```python
from build123d import *

# Parameters (mm, degrees)
PAD_DEPTH        = 1
POCKET_DEPTH     = 0.001
HOLE_D           = 1.75
HOLE_CSINK_D     = 3.3
HOLE_CSINK_ANGLE = 90
SKETCH025_R      = 5.25
SKETCH025_R_2    = 1.5
POCKET007_DEPTH  = 5
POCKET008_DEPTH  = 1.001
POCKET010_DEPTH  = 5
POCKET011_DEPTH  = 1.001


with BuildPart() as part:
    # Sketch → Pad (new body)
    with BuildSketch(Plane.XY):
        with BuildLine():
            Line((-51.8, 52.175), (51.8, 52.175))
            ThreePointArc((52.175, 51.8), (52.065165, 52.065165), (51.8, 52.175))
            Line((52.175, 51.8), (52.175, -51.8))
            ThreePointArc((51.8, -52.175), (52.065165, -52.065165), (52.175, -51.8))
            Line((51.8, -52.175), (-51.8, -52.175))
            ThreePointArc((-52.175, -51.8), (-52.065165, -52.065165), (-51.8, -52.175))
            Line((-52.175, -51.8), (-52.175, 51.8))
            ThreePointArc((-51.8, 52.175), (-52.065165, 52.065165), (-52.175, 51.8))
        make_face()
    extrude(amount=-PAD_DEPTH)

    # Sketch002 → Pocket (cut, through all)
    with BuildSketch(Plane.XY.offset(-4.8)):
        with BuildLine():
            Line((-45, 50.175), (45, 50.175))
            ThreePointArc((45, 50.175), (45.353553, 50.321447), (45.5, 50.675))
            ThreePointArc((45.5, 50.675), (45.353553, 51.028553), (45, 51.175))
            Line((-45, 51.175), (45, 51.175))
            ThreePointArc((-45, 51.175), (-45.353553, 51.028553), (-45.5, 50.675))
            ThreePointArc((-45.5, 50.675), (-45.353553, 50.321447), (-45, 50.175))
        make_face()
        with BuildLine():
            Line((-45, -51.175), (45, -51.175))
            ThreePointArc((45, -51.175), (45.353553, -51.028553), (45.5, -50.675))
            ThreePointArc((45.5, -50.675), (45.353553, -50.321447), (45, -50.175))
            Line((-45, -50.175), (45, -50.175))
            ThreePointArc((-45, -50.175), (-45.353553, -50.321447), (-45.5, -50.675))
            ThreePointArc((-45.5, -50.675), (-45.353553, -51.028553), (-45, -51.175))
        make_face()
        with BuildLine():
            Line((51.175, -45), (51.175, 45))
            ThreePointArc((51.175, 45), (51.028553, 45.353553), (50.675, 45.5))
            ThreePointArc((50.675, 45.5), (50.321447, 45.353553), (50.175, 45))
            Line((50.175, -45), (50.175, 45))
            ThreePointArc((50.175, -45), (50.321447, -45.353553), (50.675, -45.5))
            ThreePointArc((50.675, -45.5), (51.028553, -45.353553), (51.175, -45))
        make_face()
        with BuildLine():
            Line((-50.175, -45), (-50.175, 45))
            ThreePointArc((-50.175, 45), (-50.321447, 45.353553), (-50.675, 45.5))
            ThreePointArc((-50.675, 45.5), (-51.028553, 45.353553), (-51.175, 45))
            Line((-51.175, -45), (-51.175, 45))
            ThreePointArc((-51.175, -45), (-51.028553, -45.353553), (-50.675, -45.5))
            ThreePointArc((-50.675, -45.5), (-50.321447, -45.353553), (-50.175, -45))
        make_face()
    extrude(amount=-POCKET_DEPTH, mode=Mode.SUBTRACT)

    # Hole (through all)
    with Locations(Plane.XY):
        with Locations((-50, 50), (50, 50), (50, -50), (-50, -50)):
            CounterSinkHole(HOLE_D / 2, HOLE_CSINK_D / 2, counter_sink_angle=HOLE_CSINK_ANGLE)

    # Sketch025 → Pocket007 (cut)
    with BuildSketch(Plane.XY):
        with Locations((26.67, 26.67)):
            Circle(SKETCH025_R)
        with Locations((5.824921, 36.39022)):
            Circle(SKETCH025_R_2)
        with Locations((7.829503, 39.862258)):
            Circle(SKETCH025_R_2)
        with Locations((10.406544, 42.933456)):
            Circle(SKETCH025_R_2)
        with Locations((13.477742, 45.510497)):
            Circle(SKETCH025_R_2)
        with Locations((16.94978, 47.515079)):
            Circle(SKETCH025_R_2)
    extrude(amount=-POCKET007_DEPTH, mode=Mode.SUBTRACT)

    # Sketch027 → Pocket008 (cut, through all)
    with BuildSketch(Plane.XY):
        with BuildLine():
            Line((-49.17, 11.27), (-49.17, 42.07))
            ThreePointArc((-47.17, 44.07), (-48.584214, 43.484214), (-49.17, 42.07))
            Line((-47.17, 44.07), (-6.17, 44.07))
            ThreePointArc((-4.17, 42.07), (-4.755786, 43.484214), (-6.17, 44.07))
            Line((-4.17, 42.07), (-4.17, 11.27))
            ThreePointArc((-6.17, 9.27), (-4.755786, 9.855786), (-4.17, 11.27))
            Line((-6.17, 9.27), (-47.17, 9.27))
            ThreePointArc((-49.17, 11.27), (-48.584214, 9.855786), (-47.17, 9.27))
        make_face()
    extrude(amount=-POCKET008_DEPTH, mode=Mode.SUBTRACT)

    # Sketch029 → Pocket010 (cut)
    with BuildSketch(Plane.XY):
        with BuildLine():
            ThreePointArc((-33.17, 6.27), (-34.67, 4.77), (-33.17, 3.27))
            Line((-33.17, 3.27), (-30.17, 3.27))
            ThreePointArc((-30.17, 3.27), (-28.67, 4.77), (-30.17, 6.27))
            Line((-30.17, 6.27), (-33.17, 6.27))
        make_face()
        with BuildLine():
            ThreePointArc((-23.17, 6.27), (-24.67, 4.77), (-23.17, 3.27))
            Line((-23.17, 3.27), (-20.17, 3.27))
            ThreePointArc((-20.17, 3.27), (-18.67, 4.77), (-20.17, 6.27))
            Line((-20.17, 6.27), (-23.17, 6.27))
        make_face()
        with BuildLine():
            ThreePointArc((-13.17, 6.27), (-14.67, 4.77), (-13.17, 3.27))
            Line((-13.17, 3.27), (-10.17, 3.27))
            ThreePointArc((-10.17, 3.27), (-8.67, 4.77), (-10.17, 6.27))
            Line((-10.17, 6.27), (-13.17, 6.27))
        make_face()
        with BuildLine():
            ThreePointArc((-43.17, 6.27), (-44.67, 4.77), (-43.17, 3.27))
            Line((-43.17, 3.27), (-40.17, 3.27))
            ThreePointArc((-40.17, 3.27), (-38.67, 4.77), (-40.17, 6.27))
            Line((-40.17, 6.27), (-43.17, 6.27))
        make_face()
    extrude(amount=-POCKET010_DEPTH, mode=Mode.SUBTRACT)

    # Sketch030 → Pocket011 (cut, through all)
    with BuildSketch(Plane.XY):
        with BuildLine():
            Line((-48.505, -19.735), (-48.505, -6.935))
            ThreePointArc((-46.405, -4.835), (-47.889924, -5.450076), (-48.505, -6.935))
            Line((-46.405, -4.835), (-33.605, -4.835))
            ThreePointArc((-31.505, -6.935), (-32.120076, -5.450076), (-33.605, -4.835))
            Line((-31.505, -6.935), (-31.505, -19.735))
            ThreePointArc((-33.605, -21.835), (-32.120076, -21.219924), (-31.505, -19.735))
            Line((-33.605, -21.835), (-46.405, -21.835))
            ThreePointArc((-48.505, -19.735), (-47.889924, -21.219924), (-46.405, -21.835))
        make_face()
        with BuildLine():
            Line((-21.835, -19.735), (-21.835, -6.935))
            ThreePointArc((-19.735, -4.835), (-21.219924, -5.450076), (-21.835, -6.935))
            Line((-19.735, -4.835), (-6.935, -4.835))
            ThreePointArc((-4.835, -6.935), (-5.450076, -5.450076), (-6.935, -4.835))
            Line((-4.835, -6.935), (-4.835, -19.735))
            ThreePointArc((-6.935, -21.835), (-5.450076, -21.219924), (-4.835, -19.735))
            Line((-6.935, -21.835), (-19.735, -21.835))
            ThreePointArc((-21.835, -19.735), (-21.219924, -21.219924), (-19.735, -21.835))
        make_face()
        with BuildLine():
            Line((4.835, -19.735), (4.835, -6.935))
            ThreePointArc((6.935, -4.835), (5.450076, -5.450076), (4.835, -6.935))
            Line((6.935, -4.835), (19.735, -4.835))
            ThreePointArc((21.835, -6.935), (21.219924, -5.450076), (19.735, -4.835))
            Line((21.835, -6.935), (21.835, -19.735))
            ThreePointArc((19.735, -21.835), (21.219924, -21.219924), (21.835, -19.735))
            Line((19.735, -21.835), (6.935, -21.835))
            ThreePointArc((4.835, -19.735), (5.450076, -21.219924), (6.935, -21.835))
        make_face()
        with BuildLine():
            Line((31.505, -19.735), (31.505, -6.935))
            ThreePointArc((33.605, -4.835), (32.120076, -5.450076), (31.505, -6.935))
            Line((33.605, -4.835), (46.405, -4.835))
            ThreePointArc((48.505, -6.935), (47.889924, -5.450076), (46.405, -4.835))
            Line((48.505, -6.935), (48.505, -19.735))
            ThreePointArc((46.405, -21.835), (47.889924, -21.219924), (48.505, -19.735))
            Line((46.405, -21.835), (33.605, -21.835))
            ThreePointArc((31.505, -19.735), (32.120076, -21.219924), (33.605, -21.835))
        make_face()
        with BuildLine():
            Line((31.505, -46.405), (31.505, -33.605))
            ThreePointArc((33.605, -31.505), (32.120076, -32.120076), (31.505, -33.605))
            Line((33.605, -31.505), (46.405, -31.505))
            ThreePointArc((48.505, -33.605), (47.889924, -32.120076), (46.405, -31.505))
            Line((48.505, -33.605), (48.505, -46.405))
            ThreePointArc((46.405, -48.505), (47.889924, -47.889924), (48.505, -46.405))
            Line((46.405, -48.505), (33.605, -48.505))
            ThreePointArc((31.505, -46.405), (32.120076, -47.889924), (33.605, -48.505))
        make_face()
        with BuildLine():
            Line((4.835, -46.405), (4.835, -33.605))
            ThreePointArc((6.935, -31.505), (5.450076, -32.120076), (4.835, -33.605))
            Line((6.935, -31.505), (19.735, -31.505))
            ThreePointArc((21.835, -33.605), (21.219924, -32.120076), (19.735, -31.505))
            Line((21.835, -33.605), (21.835, -46.405))
            ThreePointArc((19.735, -48.505), (21.219924, -47.889924), (21.835, -46.405))
            Line((19.735, -48.505), (6.935, -48.505))
            ThreePointArc((4.835, -46.405), (5.450076, -47.889924), (6.935, -48.505))
        make_face()
        with BuildLine():
            Line((-21.835, -46.405), (-21.835, -33.605))
            ThreePointArc((-19.735, -31.505), (-21.219924, -32.120076), (-21.835, -33.605))
            Line((-19.735, -31.505), (-6.935, -31.505))
            ThreePointArc((-4.835, -33.605), (-5.450076, -32.120076), (-6.935, -31.505))
            Line((-4.835, -33.605), (-4.835, -46.405))
            ThreePointArc((-6.935, -48.505), (-5.450076, -47.889924), (-4.835, -46.405))
            Line((-6.935, -48.505), (-19.735, -48.505))
            ThreePointArc((-21.835, -46.405), (-21.219924, -47.889924), (-19.735, -48.505))
        make_face()
        with BuildLine():
            Line((-48.505, -46.405), (-48.505, -33.605))
            ThreePointArc((-46.405, -31.505), (-47.889924, -32.120076), (-48.505, -33.605))
            Line((-46.405, -31.505), (-33.605, -31.505))
            ThreePointArc((-31.505, -33.605), (-32.120076, -32.120076), (-33.605, -31.505))
            Line((-31.505, -33.605), (-31.505, -46.405))
            ThreePointArc((-33.605, -48.505), (-32.120076, -47.889924), (-31.505, -46.405))
            Line((-33.605, -48.505), (-46.405, -48.505))
            ThreePointArc((-48.505, -46.405), (-47.889924, -47.889924), (-46.405, -48.505))
        make_face()
    extrude(amount=-POCKET011_DEPTH, mode=Mode.SUBTRACT)


solid = part.part
```
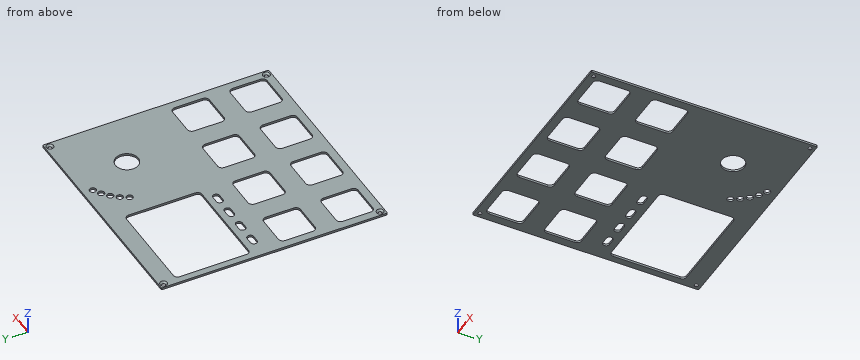
Can you work these out from the model? Positions are in its coordinate system, mm. Coordinates: 2 decimals unless noted, no trailing zeros. Order: outer loops, then holes, each group sorted by start corner. A loop starts at its lowest first (then second) coordinate and runs counter-clockwise, first axis right, second up.
1. If we section it at D-D (z = -0.6): Give the number of separate pieces and of enclosed holes in the cut face, then the cut area to 3 significant figures.
2. If we section it at A-A (y = 26.67): Please give me the cut outline in (x, z) (3 decimals).
3. I'm going to push flat-ended pins straight in: pin 1 (12 mm diameter, centred on x = -9.5, y = -23, fed in from +Z); pin 2 (2.5 mm diameter, centred on x = 50, y = 50, fed in from +Z). Where does each tip first touch, or does it pass through?
4. I need wall thicknesses on line 1 (X direction, y = -44, z = -0.5) (3 decimals); line 2 (Y direction, x = -45, z = -0.8) (3 decimals); line 3 (X direction, y = 50, z = -0.75) (3 decimals). Which ranges of each line are inside material? Lowest first, please.
5. If we section it at C-C (y = 4.77): Please give me the cut outline in (x, z) (3 decimals), then the cut area to 4 significant figures.
6. If we section it at B-B (x = 26.67): Please give me the cut outline in (y, z) (3 decimals), then the cut area to 4 significant figures.
Entries:
1. separate pieces: 1
1. enclosed holes: 23
1. area: 6,840 mm2
2. outline: (-52.175, -1) - (-49.17, -1) - (-49.17, 0) - (-52.175, 0) - close; (-4.17, -1) - (21.42, -1) - (21.42, 0) - (-4.17, 0) - close; (31.92, -1) - (52.175, -1) - (52.175, 0) - (31.92, 0) - close
3. pin 1: stops at z = 0
3. pin 2: stops at z = -0.4
4. line 1: x = -52.175 to -48.505, -31.505 to -21.835, -4.835 to 4.835, 21.835 to 31.505, 48.505 to 52.175
4. line 2: y = -52.175 to -48.505, -31.505 to -21.835, -4.835 to 9.27, 44.07 to 52.175
4. line 3: x = -52.175 to -50.9, -49.1 to 49.1, 50.9 to 52.175
5. outline: (-52.175, -1) - (-44.67, -1) - (-44.67, 0) - (-52.175, 0) - close; (-38.67, -1) - (-34.67, -1) - (-34.67, 0) - (-38.67, 0) - close; (-28.67, -1) - (-24.67, -1) - (-24.67, 0) - (-28.67, 0) - close; (-18.67, -1) - (-14.67, -1) - (-14.67, 0) - (-18.67, 0) - close; (-8.67, -1) - (52.175, -1) - (52.175, 0) - (-8.67, 0) - close
5. area: 80.35 mm2
6. outline: (-52.175, -1) - (21.42, -1) - (21.42, 0) - (-52.175, 0) - close; (31.92, -1) - (52.175, -1) - (52.175, 0) - (31.92, 0) - close
6. area: 93.85 mm2
